For this review, take the finished solid that the model builds, in its own axes (mm). Give positions to 0.01 mm unless a question says otherwise; leave off trailing zeros. Loops run counter-clockwise (first coordinate to the right, second up) from the corner with the lowest first, then second, coordinate; pieces in that order, holes last. Notation, with made-up numbers: (4, 27.5) - (54, 27.5) arc R28 ccw to (54, 53.5) - close; hole circle Ø10 at (77, 9). An arc over 180 degrees is marked (long way). Put each result on its own line as item: value.
from build123d import *


with BuildPart() as part:
    # 草图1 → 旋转1 (revolve)
    with BuildSketch(Plane(origin=(0, 0, 0), x_dir=(-1, 0, 0), z_dir=(0, 0, -1)), mode=Mode.PRIVATE) as revolve_1_sk:
        with BuildLine():
            Line((-387, 1.7), (-387, 0))
            Line((-387, 0), (0, 0))
            Line((0, 0), (0, 2.7))
            Line((0, 2.7), (-0.3, 3))
            Line((-0.3, 3), (-2.2, 3))
            Line((-2.2, 3), (-2.2, 2.85))
            Line((-2.2, 2.85), (-3, 2.85))
            Line((-3, 2.85), (-3, 3))
            Line((-3, 3), (-8.8, 3))
            ThreePointArc((-8.8, 3), (-8.941421356, 3.058578644), (-9, 3.2))
            Line((-9, 3.2), (-9, 3.7))
            Line((-9, 3.7), (-9.3, 4))
            Line((-9.3, 4), (-348.7, 4))
            Line((-348.7, 4), (-349, 3.7))
            Line((-349, 3.7), (-349, 3.2))
            ThreePointArc((-349, 3.2), (-349.058578644, 3.058578644), (-349.2, 3))
            Line((-349.2, 3), (-378.7, 3))
            Line((-378.7, 3), (-379, 2.7))
            Line((-379, 2.7), (-379, 2.2))
            ThreePointArc((-379, 2.2), (-379.058578644, 2.058578644), (-379.2, 2))
            Line((-379.2, 2), (-386.7, 2))
            Line((-386.7, 2), (-387, 1.7))
        make_face()
    revolve(revolve_1_sk.sketch.rotate(Axis((387, 0, 0), (-1, 0, 0)), 180), axis=Axis((387, 0, 0), (-1, 0, 0)))


solid = part.part
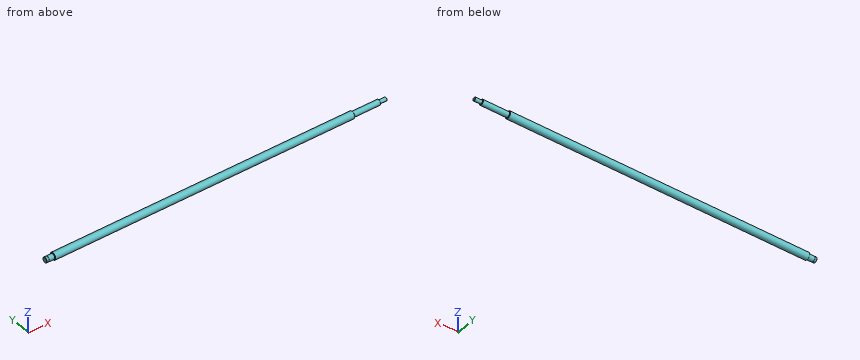
1) Wall thickness on line 1 (X direction, y = 3, z = -1.5); line 2 (X direction, y = -2, z = -1.5); line 3 (Z direction, x = 41, y = 3): over which ranges is each line inside the solid? List them lowest first.
Geometry check:
line 1: x = 9 to 349
line 2: x = 0 to 379
line 3: z = -2.65 to 2.65
2) Take a section at B-B on x = 358.5. State the section outline as (y, z) points.
Geometry check:
outline: circle Ø6 at (0, 0)
3) Take a section at A-A on x = 27.5. State the section outline as (y, z) points, and give its area (3 significant figures).
Geometry check:
outline: circle Ø8 at (0, 0)
area: 50.3 mm²
